```python
from build123d import *

# Parameters (mm, degrees)
SKETCH2_W  = 19.05
SKETCH2_H  = 3.4036
SLOT_DEPTH = 4.9022


with BuildPart() as part:
    # BodySke → BaseBody (revolve)
    with BuildSketch(Plane.XY):
        with BuildLine():
            Line((2.552216058, 9.525), (47.157428837, 9.525))
            ThreePointArc((47.157428837, 9.525), (49.8582952, 5.098871191), (50.8, 0))
            Line((50.8, 0), (0, 0))
            ThreePointArc((0, 0), (0.649113009, 4.930502809), (2.552216058, 9.525))
        make_face()
    revolve(axis=Axis((-12.7, 0, 0), (1, 0, 0)))

    # Sketch2 → Slot (cut)
    with BuildSketch(Plane(origin=(0, 0, 0), x_dir=(0, 0, -1), z_dir=(1, 0, 0))):
        Rectangle(SKETCH2_W, SKETCH2_H)
    extrude(amount=SLOT_DEPTH, mode=Mode.SUBTRACT)


solid = part.part
```
Source: CAD feature listing. Evaluate the final solid. Frame: model axes, mm. Round coordinates to 2 decimals unless told otherwise and drop trailing zeros. Write each loop counter-clockwise with the first axis right and the second up, starting at its lowest first coordinate (ties: lowest second). Pieces come first, ordered by that corner, then holes. Notation, with made-up numbers: M 85.5,21 L 95.5,21 A18 cw 95.5,33 Z; hole C 20.25,24.25 d5. An arc over 180 degrees is marked long. Use CSV: the item, a comma, the result in double quotes. Start each with the question number.
Q1. Cut plane D-D on z = 7. Output: boundary loops of the cut face in (x, y).
Q2. Line query: line 1 (Z direction, x = 42, y = -0.25); line 2 (Y direction, x = 12, z = 1.75). Output: solid intervals per line, ascending. Write a range as from..to.
Q3. First-contact query: P1, Ø4, axis at x = 3.5, z = -1.5, coming from the -Y side (3 decimals); P2, Ø2, axis at x = 15.5, y = -1.5, coming from the -Z side; P3, Ø1.5, axis at x = 16, y = -5.5, coming from the -Z side; P4, Ø4, axis at y = 0.5, z = 3, coming from the -X side. Flat tips, straight axial feed; report the tip coordinate or a pass-through.
Q4. Cut plane A-A on z = 0. Output: boundary loops of the cut face in (x, y) (3 decimals), plus the area to 3 significant figures.
Q5. Cut plane C-C on x = 44.5. Output: boundary loops of the cut face in (y, z) (3 decimals).
Q6. Pull-direction query (Y, two-part tool) for faces 1 (the face through (25.167, -7.559, -5.796)), 2 (the face through (4.902, 0, 0)), 3 (the face through (3, 1.702, 0)); classes: +Y half, -Y half, draft (parallel to the pull), parting line (faces both ways), or undercut.
Q7. Cut plane B-B on y = 0. Output: boundary loops of the cut face in (x, z) (3 decimals).
Results found:
1,outline,"M 1.41,-1.7 A17.72 ccw 2.55,-6.46 L 47.16,-6.46 A12.44 ccw 47.16,6.46 L 2.55,6.46 A17.72 ccw 1.41,1.7 L 4.9,1.7 L 4.9,-1.7 Z"
2,line 1,"-9.52..9.52"
2,line 2,"-9.36..9.36"
3,P1,"y = -9.525"
3,P2,"z = -9.51"
3,P3,"z = -8.26"
3,P4,"x = 0.13"
4,outline,"M 0.076,-1.702 A19.05 ccw 2.552,-9.525 L 47.157,-9.525 A14.275 ccw 47.157,9.525 L 2.552,9.525 A19.05 ccw 0.076,1.702 L 4.902,1.702 L 4.902,-1.702 Z"
4,area,"914 mm^2"
5,outline,"C 0,0 d19.05"
6,face 1,"parting line"
6,face 2,"undercut"
6,face 3,"undercut"
7,outline,"M 4.902,-9.525 L 47.157,-9.525 A14.275 ccw 47.157,9.525 L 4.902,9.525 Z"
